```python
from build123d import *

# Parameters (mm, degrees)
F1_DEPTH = 25.4
F2_R     = 2.394714
F2_R_2   = 2.525122
F2_R_3   = 2.568066
F3_DEPTH = 25.4


with BuildPart() as f1:
    # F0 (on Front) → F1 (new body)
    with BuildSketch(Plane.XZ):
        with BuildLine():
            Line((7.943742, 14.15978), (-4.756258, 14.15978))
            ThreePointArc((-4.756258, 14.15978), (-9.246386, 12.299908), (-11.106258, 7.80978))
            Line((-11.106258, 7.80978), (-11.106258, -4.89022))
            ThreePointArc((-11.106258, -4.89022), (-9.246386, -9.380348), (-4.756258, -11.24022))
            Line((-4.756258, -11.24022), (7.943742, -11.24022))
            ThreePointArc((7.943742, -11.24022), (12.43387, -9.380348), (14.293742, -4.89022))
            Line((14.293742, -4.89022), (14.293742, 7.80978))
            ThreePointArc((14.293742, 7.80978), (12.43387, 12.299908), (7.943742, 14.15978))
        make_face()
    extrude(amount=F1_DEPTH)

    # F2 (on face) → F3 (cut)
    with BuildSketch(Plane.XZ.offset(25.4)):
        with Locations((-5.862328, 8.878076)):
            Circle(F2_R)
        with Locations((0, 8.878076)):
            Circle(F2_R_2)
        with Locations((7.943742, 7.80978)):
            Circle(F2_R_3)
    extrude(amount=-F3_DEPTH, mode=Mode.SUBTRACT)


solid = f1.part
```
Design review of the part built by this model. Coordinates are the model's own, in mm. Round coordinates to 2 decimals unless told otherwise and drop trailing zeros. Write each loop counter-clockwise with the first axis right and the second up, starting at its lowest first coordinate (ties: lowest second). Pieces come first, ordered by that corner, then holes.
Item 1: We need section B-B on z = 10. Write out the cut boundary in (x, y), and give its area (3 significant figures).
Item 2: For probe 1 along Z at (x, y) = (0, -19.5); probe 2 along X at (y, z) = (-8.5, 7.25); probe 3 along X at (y, z) = (-19.25, 9), list the stretches that pass through material, from the lowest coordinate up.
Item 3: We need section D-D on x = 7.25. Write out the cut boundary in (y, z).
Item 4: The part is to be moulded in two halves that separate along Z. For faces 1 (the cylindrical face through (12.384, -12.522, -9.429)), 2 (the cylindrical face through (-6.38, -12.88, 6.54)), 3 (the flat face through (1, 0, 2)), say which applies: +Z half, -Z half, draft (parallel to the pull), parting line (faces both ways), or undercut.
Item 5: Clearance check with a flat-ended pin moving along its axis: pin 1 Ø1.5 at (x, z) = (8.5, 8.5) entering from +Y. State where the tip first meets the part, or that it passes through.
Item 6: We need section C-C on y = -22. Write out the cut boundary in (x, z), and give its area (3 significant figures).
Item 7: We need section A-A on x = 0. Write out the cut boundary in (y, z), and give its area (3 significant figures).
Returned:
1. outline: (-10.72, -25.4) - (-7.98, -25.4) - (-7.98, 0) - (-10.72, 0) - close; (-3.75, -25.4) - (-2.26, -25.4) - (-2.26, 0) - (-3.75, 0) - close; (2.26, -25.4) - (6.6, -25.4) - (6.6, 0) - (2.26, 0) - close; (9.28, -25.4) - (13.9, -25.4) - (13.9, 0) - (9.28, 0) - close
1. area: 335 mm2
2. probe 1: z = -11.24 to 6.35, 11.4 to 14.16
2. probe 2: x = -11.11 to -7.62, -4.11 to -1.93, 1.93 to 5.44, 10.45 to 14.29
2. probe 3: x = -10.99 to -8.25, -3.47 to -2.52, 2.52 to 5.67, 10.22 to 14.18
3. outline: (-25.4, -11.24) - (0, -11.24) - (0, 5.34) - (-25.4, 5.34) - close; (-25.4, 10.28) - (0, 10.28) - (0, 14.16) - (-25.4, 14.16) - close
4. face 1: -Z half
4. face 2: undercut
4. face 3: draft
5. pin 1: passes through
6. outline: (-11.11, -4.89) arc R6.35 ccw to (-4.76, -11.24) - (7.94, -11.24) arc R6.35 ccw to (14.29, -4.89) - (14.29, 7.81) arc R6.35 ccw to (7.94, 14.16) - (-4.76, 14.16) arc R6.35 ccw to (-11.11, 7.81) - close; hole circle Ø4.79 at (-5.86, 8.88); hole circle Ø5.05 at (0, 8.88); hole circle Ø5.14 at (7.94, 7.81)
6. area: 552 mm2
7. outline: (-25.4, -11.24) - (0, -11.24) - (0, 6.35) - (-25.4, 6.35) - close; (-25.4, 11.4) - (0, 11.4) - (0, 14.16) - (-25.4, 14.16) - close
7. area: 517 mm2
